Autodesk Inventor part; units mm, degrees
ref_plane "YZ Plane" through (0, 0, 0) normal (1, 0, 0) x (0, 1, 0)
ref_plane "XZ Plane" through (0, 0, 0) normal (0, 1, 0) x (-1, 0, 0)
ref_plane "XY Plane" through (0, 0, 0) normal (0, 0, 1) x (1, 0, 0)
sketch "Szkic1" plane through (0, 0, 0) normal (0, 1, 0) x (-1, 0, 0)
  line L0 (-6, -17.5) -> (6, -17.5)
  line L1 (6, -17.5) -> (6, 17.5)
  line L2 (6, 17.5) -> (-6, 17.5)
  line L3 (-6, 17.5) -> (-6, -17.5)
  line L4 (-6, -17.5) -> (6, 17.5) construction
  line L5 (6, -17.5) -> (-6, 17.5) construction
  circle A0 centre (0, 12.5) radius 1.75
  circle A1 centre (0, -12.5) radius 1.75
  point P0 (0, 0)
  dimension "d0" = 12
  dimension "d1" = 35
  dimension "d2" = 3.5
  dimension "d3" = 3.5
extrude "Wyciągnięcie proste1" add sketch "Szkic1" along normal blind 12
sketch "Szkic2" plane through (6, 0, 17.5) normal (1, 0, 0) x (0, 0, -1)
  arc A0 (25.5, 0) -> (9.5, 0) centre (17.5, 0) ccw
  line L0 (9.5, 0) -> (11.5, 0)
  line L1 (23.5, 0) -> (25.5, 0)
  arc A1 (23.5, 0) -> (11.5, 0) centre (17.5, 0) ccw
  dimension "d7" = 16
extrude "Wyciągnięcie proste2" cut sketch "Szkic2" against normal blind 3
sketch "Szkic3" plane through (6, 0, 6) normal (1, 0, 0) x (0, 0, -1)
  line L0 (0, 0) -> (12, 0)
  arc A0 (12, 0) -> (0, 0) centre (6, 0) ccw
extrude "Wyciągnięcie proste3" cut sketch "Szkic3" against normal blind 9
sketch "Szkic4" plane through (-6, 0, -17.5) normal (-1, 0, 0) x (0, 0, 1)
  arc A0 (25.5, 0) -> (9.5, 0) centre (17.5, 0) ccw
  line L0 (25.5, 0) -> (9.5, 0)
  dimension "d13" = 16
sketch "Szkic5" plane through (-6, 0, -17.5) normal (-1, 0, 0) x (0, 0, 1)
  point P0 (17.5, 0)
extrude "Wyciągnięcie proste4" cut sketch "Szkic4" against normal blind 3
sketch "Szkic6" plane through (0, 12, 0) normal (0, 1, 0) x (1, 0, 0)
  circle A0 centre (0, -12.5) radius 2.5
  circle A1 centre (0, 12.5) radius 2.5
  point P0 (0, 0)
  dimension "d16" = 5
  dimension "d17" = 5
extrude "Wyciągnięcie proste5" cut sketch "Szkic6" against normal blind 2
chamfer "Faza1" distance 12 distance2 3 1 edges at (6, 6, 17.5) measured on face at (-2, 4, 17.5)
properties part number "ExtruderClamp"
Geometry check sheet. Reference: the model listing, model coordinates, mm. A direction names the side the tool comes from. Give positions to 0.01 mm unless a question says otherwise; leave off trailing zeros. Write each loop counter-clockwise with the first axis right and the second up, starting at its lowest first coordinate (ties: lowest second). Pieces come first, ordered by that corner, then holes. Notation, with made-up numbers: (16.5, -27) -> (45.5, -27) arc R22 ccw to (45.5, -17) -> close; hole circle Ø11 at (-3, -38.5). An arc over 180 degrees is marked (long way). One line per question, with ' | ' between items.
Item 1: Scan lines: line 1 along X through (y, z) = (7.5, 12.5); line 2 along Z through (x, y) = (0, 10.95); line 3 along Z through (x, y) = (-1.5, 10.75). Record each from-to range of solid material in increasing order.
Determined:
line 1: -6 to -1.75, 1.75 to 6 | line 2: -17.5 to -15, -10 to 10, 15 to 16 | line 3: -17.5 to -14.5, -10.5 to 10.5, 14.5 to 16.38
Item 2: Sectioned sample at B-B, the plane z = -12.5. Record the boundary of the cut face in (x, y).
Determined:
outline: (-6, 0) -> (-1.75, 0) -> (-1.75, 10) -> (-2.5, 10) -> (-2.5, 12) -> (-6, 12) -> close; (1.75, 0) -> (6, 0) -> (6, 12) -> (2.5, 12) -> (2.5, 10) -> (1.75, 10) -> close
Item 3: Draft check along Z on faces 6 (the flat face through (0, 6, 16)), 7 (the flat face through (0, 0, -10)), 8 (the flat face through (-3, 7, 0)). Enter one of: released by +Z, released by -Z, zero draft, split by the parting line, or undercut.
Determined:
face 6: released by +Z | face 7: zero draft | face 8: undercut
Item 4: Access from +Z, -Z, +X, -X, +Y, -Y to the whole of each face (thin tool, end or side, straight path). Record for faces 1 (the flat face through (0, 6, -17.5)), 2 (the flat face through (3, 7, 0)), 3 (the cylindrical face through (-0.54, 11.01, 14.94)), 4 (the cylindrical face through (0.228, 4.93, 10.765)), 5 (the cylindrical face through (-5, 8, 0)).
Determined:
face 1: -Z, +X, -X, +Y, -Y | face 2: +X, -Y | face 3: +Y | face 4: +Y, -Y | face 5: -X, -Y
Item 5: Sectioned sample at C-C, the plane x = 0. Record the boundary of the cut face in (y, z).
Determined:
outline: (0, -17.5) -> (12, -17.5) -> (12, -15) -> (10, -15) -> (10, -14.25) -> (0, -14.25) -> close; (0, -10.75) -> (10, -10.75) -> (10, -10) -> (12, -10) -> (12, 10) -> (10, 10) -> (10, 10.75) -> (0, 10.75) -> (0, 6) arc R6 cw to (0, -6) -> close; (0, 14.25) -> (10, 14.25) -> (10, 15) -> (12, 15) -> (12, 16) -> (0, 16) -> close
Item 6: Sectioned sample at A-A, the plane y = 3.75. State how many separate pieces and enclosed holes the cut face has, plus the area to 3 significant figures.
Determined:
separate pieces: 2 | enclosed holes: 2 | area: 242 mm^2
Item 7: Depth check by flat-ended pin: pin 1 (6 mm diameter, centred on x = -1.5, y = 5, fed in from +Z); pin 2 (4 mm diameter, centred on x = 0, z = -12.5, fed in from +Y); pin 3 (6 mm diameter, centred on y = 2, z = -3, fed in from +X). Enter the tip coordinate at first touch or a pass-through.
Determined:
pin 1: z = 17.13 | pin 2: y = 10 | pin 3: x = 3
